from build123d import *

# Parameters (mm, degrees)
BOSS_EXTRUDE1_DEPTH = 3
CUT_EXTRUDE1_REACH  = 169.024
SKETCH3_R           = 1.1
CUT_EXTRUDE2_REACH  = 169.024
SKETCH5_R           = 3.4
CUT_EXTRUDE3_REACH  = 169.024
SKETCH7_R           = 1.5
BOSS_EXTRUDE3_DEPTH = 3
FILLET1_R           = 2
SKETCH8_R           = 5
BOSS_EXTRUDE4_DEPTH = 3
CUT_EXTRUDE4_REACH  = 169.024
SKETCH9_R           = 1.5
FILLET2_R           = 5
CUT_EXTRUDE5_REACH  = 169.024
SKETCH10_R          = 1.5


with BuildPart() as part:
    # Sketch1 → Boss-Extrude1 (new body)
    with BuildSketch(Plane(origin=(-22.718758449, 0, 0), x_dir=(0, 0, -1), z_dir=(1, 0, 0))):
        with BuildLine():
            Line((33.252275896, 149.750258484), (43.222646201, 20.519489254))
            ThreePointArc((43.222646201, 20.519489254), (20.789313015, -3.711279977), (-1.644020172, 20.519489254))
            Line((-1.644020172, 20.519489254), (8.326350133, 149.750258484))
            ThreePointArc((8.326350133, 149.750258484), (20.789313015, 161.288720023), (33.252275896, 149.750258484))
        make_face()
    extrude(amount=BOSS_EXTRUDE1_DEPTH)

    # Sketch3 → Cut-Extrude1 (cut, up to next)
    with BuildSketch(Plane(origin=(-19.718758449, 0, 0), x_dir=(0, 0, -1), z_dir=(1, 0, 0)), mode=Mode.PRIVATE) as cut_extrude1_sk1:
        with Locations((20.789313015, 157.538720023)):
            Circle(SKETCH3_R)
    cut_extrude1_tool1 = extrude(cut_extrude1_sk1.sketch, amount=-CUT_EXTRUDE1_REACH, mode=Mode.PRIVATE) & part.part
    # Sketch3 → Cut-Extrude1 (cut, up to next)
    with BuildSketch(Plane(origin=(-19.718758449, 0, 0), x_dir=(0, 0, -1), z_dir=(1, 0, 0)), mode=Mode.PRIVATE) as cut_extrude1_sk2:
        with Locations((20.789313015, 129.738720023)):
            Circle(SKETCH3_R)
    cut_extrude1_tool2 = extrude(cut_extrude1_sk2.sketch, amount=-CUT_EXTRUDE1_REACH, mode=Mode.PRIVATE) & part.part
    # Sketch3 → Cut-Extrude1 (cut, up to next)
    with BuildSketch(Plane(origin=(-19.718758449, 0, 0), x_dir=(0, 0, -1), z_dir=(1, 0, 0)), mode=Mode.PRIVATE) as cut_extrude1_sk3:
        with BuildLine():
            Line((14.689313015, 154.038720023), (14.689313015, 148.788720023))
            Line((14.689313015, 148.788720023), (14.689313015, 133.238720023))
            ThreePointArc((14.689313015, 133.238720023), (14.938272251, 132.637679259), (15.539313015, 132.388720023))
            Line((15.539313015, 132.388720023), (26.039313015, 132.388720023))
            ThreePointArc((26.039313015, 132.388720023), (26.640353779, 132.637679259), (26.889313015, 133.238720023))
            Line((26.889313015, 133.238720023), (26.889313015, 148.788720023))
            Line((26.889313015, 148.788720023), (26.889313015, 154.038720023))
            ThreePointArc((26.889313015, 154.038720023), (26.640353779, 154.639760787), (26.039313015, 154.888720023))
            Line((26.039313015, 154.888720023), (20.789313015, 154.888720023))
            Line((20.789313015, 154.888720023), (15.539313015, 154.888720023))
            ThreePointArc((15.539313015, 154.888720023), (14.938272251, 154.639760787), (14.689313015, 154.038720023))
        make_face()
    cut_extrude1_tool3 = extrude(cut_extrude1_sk3.sketch, amount=-CUT_EXTRUDE1_REACH, mode=Mode.PRIVATE) & part.part
    add(cut_extrude1_tool1.solids().sort_by_distance((-19.718758, 157.53872, -20.789313))[0], mode=Mode.SUBTRACT)
    add(cut_extrude1_tool2.solids().sort_by_distance((-19.718758, 129.73872, -20.789313))[0], mode=Mode.SUBTRACT)
    add(cut_extrude1_tool3.solids().sort_by_distance((-19.718758, 143.63872, -20.789313))[0], mode=Mode.SUBTRACT)

    # Sketch5 → Cut-Extrude2 (cut, up to next)
    with BuildSketch(Plane(origin=(-19.718758449, 0, 0), x_dir=(0, 0, -1), z_dir=(1, 0, 0)), mode=Mode.PRIVATE) as cut_extrude2_sk1:
        with Locations((20.789313015, 18.788720023)):
            Circle(SKETCH5_R)
    cut_extrude2_tool1 = extrude(cut_extrude2_sk1.sketch, amount=-CUT_EXTRUDE2_REACH, mode=Mode.PRIVATE) & part.part
    add(cut_extrude2_tool1.solids().sort_by_distance((-19.718758, 18.78872, -20.789313))[0], mode=Mode.SUBTRACT)

    # Sketch6 → Cut-Extrude3 (cut, up to next)
    with BuildSketch(Plane.ZY.offset(22.718758449), mode=Mode.PRIVATE) as cut_extrude3_sk1:
        with BuildLine():
            Line((-12.212541883, 109.452410499), (-7.597239032, 49.809553356))
            ThreePointArc((-7.597239032, 49.809553356), (-20.789313015, 35.557207763), (-33.981386998, 49.809553356))
            Line((-33.981386998, 49.809553356), (-29.366084146, 109.452410499))
            ThreePointArc((-29.366084146, 109.452410499), (-20.789313015, 117.391131783), (-12.212541883, 109.452410499))
        make_face()
    cut_extrude3_tool1 = extrude(cut_extrude3_sk1.sketch, amount=-CUT_EXTRUDE3_REACH, mode=Mode.PRIVATE) & part.part
    add(cut_extrude3_tool1.solids().sort_by_distance((-22.718758, 73.705728, -20.789313))[0], mode=Mode.SUBTRACT)

    # Sketch7 → Boss-Extrude3 (add)
    with BuildSketch(Plane.ZY.offset(22.718758449)):
        with BuildLine():
            Line((-32.072781677, 74.474169773), (-25.37188871, 74.474169773))
            ThreePointArc((-25.37188871, 74.474169773), (-20.789313015, 71.474169773), (-16.20673732, 74.474169773))
            Line((-16.20673732, 74.474169773), (-9.505844352, 74.474169773))
            Line((-9.505844352, 74.474169773), (-9.815373645, 78.474169773))
            Line((-9.815373645, 78.474169773), (-16.20673732, 78.474169773))
            ThreePointArc((-16.20673732, 78.474169773), (-20.789313015, 81.474169773), (-25.37188871, 78.474169773))
            Line((-25.37188871, 78.474169773), (-31.763252384, 78.474169773))
            Line((-31.763252384, 78.474169773), (-32.072781677, 74.474169773))
        make_face()
        with Locations((-20.789313015, 76.474169773)):
            Circle(SKETCH7_R, mode=Mode.SUBTRACT)
    extrude(amount=-BOSS_EXTRUDE3_DEPTH)

    # Fillet1
    fillet1_edges = [part.edges().sort_by_distance(p)[0] for p in [
        (-21.218758449, 74.474169773, -32.072781677),
        (-21.218758449, 78.474169773, -31.763252384),
        (-21.218758449, 78.474169773, -25.37188871),
        (-21.218758449, 78.474169773, -16.20673732),
        (-21.218758449, 78.474169773, -9.815373645),
        (-21.218758449, 74.474169773, -9.505844352),
        (-21.218758449, 74.474169773, -16.20673732),
        (-21.218758449, 74.474169773, -25.37188871),
    ]]
    fillet(fillet1_edges, radius=FILLET1_R)

    # Sketch8 → Boss-Extrude4 (add)
    with BuildSketch(Plane.ZY.offset(22.718758449)):
        with Locations((0.944018077, 12.965291508)):
            Circle(SKETCH8_R)
    extrude(amount=-BOSS_EXTRUDE4_DEPTH)

    # Sketch9 → Cut-Extrude4 (cut, up to next)
    with BuildSketch(Plane.ZY.offset(22.718758449), mode=Mode.PRIVATE) as cut_extrude4_sk1:
        with Locations((0.944018077, 12.965291508)):
            Circle(SKETCH9_R)
    cut_extrude4_tool1 = extrude(cut_extrude4_sk1.sketch, amount=-CUT_EXTRUDE4_REACH, mode=Mode.PRIVATE) & part.part
    add(cut_extrude4_tool1.solids().sort_by_distance((-22.718758, 12.965292, 0.944018))[0], mode=Mode.SUBTRACT)

    # Fillet2
    fillet2_edges = [part.edges().sort_by_distance(p)[0] for p in [
        (-21.218758449, 17.908803886, 1.693474793),
        (-21.218758449, 8.309355847, -0.878689557),
    ]]
    fillet(fillet2_edges, radius=FILLET2_R)

    # Sketch10 → Cut-Extrude5 (cut, up to next)
    with BuildSketch(Plane.ZY.offset(22.718758449), mode=Mode.PRIVATE) as cut_extrude5_sk1:
        with Locations((-20.789313015, 29.288720023)):
            Circle(SKETCH10_R)
    cut_extrude5_tool1 = extrude(cut_extrude5_sk1.sketch, amount=-CUT_EXTRUDE5_REACH, mode=Mode.PRIVATE) & part.part
    # Sketch10 → Cut-Extrude5 (cut, up to next)
    with BuildSketch(Plane.ZY.offset(22.718758449), mode=Mode.PRIVATE) as cut_extrude5_sk2:
        with Locations((-20.789313015, 5.288720023)):
            Circle(SKETCH10_R)
    cut_extrude5_tool2 = extrude(cut_extrude5_sk2.sketch, amount=-CUT_EXTRUDE5_REACH, mode=Mode.PRIVATE) & part.part
    add(cut_extrude5_tool1.solids().sort_by_distance((-22.718758, 29.28872, -20.789313))[0], mode=Mode.SUBTRACT)
    add(cut_extrude5_tool2.solids().sort_by_distance((-22.718758, 5.28872, -20.789313))[0], mode=Mode.SUBTRACT)


solid = part.part
Geometry: final body of the model. Coordinates: model frame, mm. A direction names the side the tool comes from. Round coordinates to 2 decimals unless told otherwise and drop trailing zeros. Loops run counter-clockwise (first coordinate to the right, second up) from the corner with the lowest first, then second, coordinate; pieces in that order, holes last. Notation, with made-up numbers: M 47.5,39 L 96.5,39 A14 cw 96.5,46 Z; hole C -12,5 d6. An arc over 180 degrees is marked long. One line per question, with ' | ' between items.
(1) Access query for faces 4 (the cylindrical face through (-21.24, 35.56, -20.48)), 5 (the flat face through (-19.719, 62, -8)). Directions: +Z, -Z, +X, -X, +Y, -Y. A direction counts if a zero-diameter tool reaches every point of the face in a straight line with its end or side. Return the directions, or none.
Check result:
face 4: +X, -X | face 5: +Z, -Z, +X, +Y, -Y
(2) Contact query for flat-ended pins moving along their axis: P1, Ø1.5, axis at x = -20.5, z = -19.5, coming from the -Y side; P2, Ø1.5, axis at x = -21, y = 142.5, coming from the -Z side; P3, Ø0.9, axis at x = -21.5, z = -22.5, coming from the +Y side (3 decimals). Output: stop coordinate, or through.
Check result:
P1: stops at y = -3.7 | P2: stops at z = -33.87 | P3: stops at y = 161.225
(3) Cut plane D-D on z = -38.5. Return the cut outline in (x, y).
Check result:
outline: M -22.72,4.91 L -19.72,4.91 L -19.72,81.73 L -22.72,81.73 Z
(4) Cut plane C-C on x = -21.4. Give the number of separate pieces and of enclosed holes in the cut face, plus the area to 3 significant figures.
Check result:
separate pieces: 1 | enclosed holes: 10 | area: 3,730 mm2
(5) Cut plane B-B on y = 51.5. Return the cut outline in (x, z), plus the area to 3 significant figures.
Check result:
outline: M -22.72,-40.83 L -19.72,-40.83 L -19.72,-33.85 L -22.72,-33.85 Z; M -22.72,-7.73 L -19.72,-7.73 L -19.72,-0.75 L -22.72,-0.75 Z | area: 41.9 mm2
(6) Cut plane A-A on y = 97.5. Return the cut outline in (x, z), plus the area to 3 significant figures.
Check result:
outline: M -22.72,-37.28 L -19.72,-37.28 L -19.72,-30.29 L -22.72,-30.29 Z; M -22.72,-11.29 L -19.72,-11.29 L -19.72,-4.3 L -22.72,-4.3 Z | area: 42.0 mm2
(7) Material intervals for line 1 along Y through (x, z) = (-21.4, -18); line 2 along Y through (x, z) = (-21.75, -23.5); line 3 along Y through (x, z) = (-22.15, -26.5), sorted ascending. Write a range as from..to.
Check result:
line 1: y = -3.54..16.84, 20.73..35.85, 72.32..80.62, 116.93..132.39, 154.89..160.97 | line 2: y = -3.55..16.74, 20.84..35.84, 72.27..80.68, 116.95..132.39, 154.89..160.99 | line 3: y = -2.97..36.85, 74.47..78.47, 115.22..132.52, 154.75..159.91
(8) Pull-direction query (Y, two-part tool) for faces 1 (the flat face through (-21.24, 84.384, -3.283)), 2 (the cylindrical face through (-21.24, 11.59, 5.75)), 3 (the cylindrical face through (-21.24, 77.96, -20.98)); classes: +Y half, -Y half, draft (parallel to the pull), parting line (faces both ways), or undercut.
Check result:
face 1: +Y half | face 2: parting line | face 3: undercut
